from build123d import *

# Parameters (mm, degrees)
CYLINDER016_R     = 1.65
CYLINDER016_DEPTH = 50
CYLINDER017_R     = 3.25
CYLINDER017_DEPTH = 2.5
BOX005_W          = 80
BOX005_H          = 100
BOX005_DEPTH      = 9.5
CYLINDER014_R     = 22.95
CYLINDER014_DEPTH = 27
CYLINDER015_R     = 27.75
CYLINDER015_DEPTH = 40
SKETCH013_R       = 27.75
PAD001_DEPTH      = 10
SKETCH014_W       = 24
SKETCH014_H       = 14.2
POCKET013_DEPTH   = 28
SKETCH015_R       = 8.1
POCKET014_DEPTH   = 15
POCKET015_DEPTH   = 14.4
PAD003_DEPTH      = 5
PAD004_DEPTH      = 10
POCKET017_DEPTH   = 10
SKETCH022_R       = 2.6
POCKET018_DEPTH   = 4.2
SKETCH023_W       = 108.293205
SKETCH023_H       = 87.132465
POCKET019_DEPTH   = 20
SKETCH024_R       = 27.699707
PAD005_DEPTH      = 10
SKETCH025_W       = 11.3
SKETCH025_H       = 5.3
POCKET020_DEPTH   = 33
POCKET021_DEPTH   = 5.3
SKETCH027_R       = 4.253317
POCKET022_DEPTH   = 8


with BuildPart() as cylinder016:
    # Cylinder016 → Cylinder016 (new body)
    with BuildSketch(Plane(origin=(0, 50, 20), x_dir=(1, 0, 0), z_dir=(0, -1, 0))):
        Circle(CYLINDER016_R)
    extrude(amount=CYLINDER016_DEPTH)


with BuildPart() as cylinder017:
    # Cylinder017 → Cylinder017 (new body)
    with BuildSketch(Plane(origin=(0, 27.75, 20), x_dir=(1, 0, 0), z_dir=(0, -1, 0))):
        Circle(CYLINDER017_R)
    extrude(amount=CYLINDER017_DEPTH)


with BuildPart() as obj1:
    # Box005 → Box005 (new body)
    with BuildSketch(Plane(origin=(-40, 0, -1), x_dir=(1, 0, 0), z_dir=(0, 0, 1))):
        with Locations((40, 50)):
            Rectangle(BOX005_W, BOX005_H)
    extrude(amount=BOX005_DEPTH)


with BuildPart() as fusion007:
    # Cylinder014 → Cylinder014 (new body)
    with BuildSketch(Plane.XY.offset(-1)):
        Circle(CYLINDER014_R)
    extrude(amount=CYLINDER014_DEPTH)

    # Cut011: cut obj1
    add(obj1.part, mode=Mode.SUBTRACT)

    # Fusion007: union Cylinder016, Cylinder017
    add(cylinder016.part)
    add(cylinder017.part)


with BuildPart() as obj2:
    # Cylinder015 → Cylinder015 (new body)
    with BuildSketch(Plane.XY.offset(-14)):
        Circle(CYLINDER015_R)
    extrude(amount=CYLINDER015_DEPTH)

    # Cut010: cut Fusion007
    add(fusion007.part, mode=Mode.SUBTRACT)

    # Sketch013 (on Face2 of BaseFeature003) → Pad001 (new body)
    with BuildSketch(Plane(origin=(0, 0, -14), x_dir=(1, 0, 0), z_dir=(0, 0, -1))):
        Circle(SKETCH013_R)
    extrude(amount=PAD001_DEPTH)

    # Sketch014 → Pocket013 (cut)
    with BuildSketch(Plane(origin=(0, 28, 0), x_dir=(-1, 0, 0), z_dir=(0, 1, 0))):
        with Locations((0, -12.1)):
            Rectangle(SKETCH014_W, SKETCH014_H)
    extrude(amount=-POCKET013_DEPTH, mode=Mode.SUBTRACT)

    # Sketch015 (on Face6 of Pocket013) → Pocket014 (cut)
    with BuildSketch(Plane(origin=(0, 0, -24), x_dir=(1, 0, 0), z_dir=(0, 0, -1))):
        Circle(SKETCH015_R)
    extrude(amount=-POCKET014_DEPTH, mode=Mode.SUBTRACT)

    # Sketch016 (on Face6 of Pocket014) → Pocket015 (cut)
    with BuildSketch(Plane(origin=(0, 0, -19.3), x_dir=(1, 0, 0), z_dir=(0, 0, -1))):
        Polygon((0, -14.036056), (12.155581, -7.018028), (12.155581, 7.018028), (0, 14.036056), (-12.155581, 7.018028), (-12.155581, -7.018028), align=None)
    extrude(amount=-POCKET015_DEPTH, mode=Mode.SUBTRACT)

    # Sketch019 (on Face8 of Pocket015) → Pad003 (join)
    with BuildSketch(Plane.XY.offset(25)):
        with BuildLine():
            ThreePointArc((-15.553331, -22.846971), (0.028426, -27.638548), (15.600294, -22.814929))
            Line((15.600294, -22.814929), (5.918583, -80.985076))
            ThreePointArc((-5.919268, -80.980951), (-0.002091, -86), (5.918583, -80.985076))
            Line((-15.553331, -22.846971), (-5.919268, -80.980951))
        make_face()
    extrude(amount=-PAD003_DEPTH)

    # Sketch020 (on Face12 of Pad003) → Pad004 (join)
    with BuildSketch(Plane.XY.offset(25)):
        with BuildLine():
            ThreePointArc((-5.898869, -81.096969), (0.071542, -85.999573), (5.92335, -80.955994))
            Line((11.272496, -48.593121), (5.92335, -80.955994))
            ThreePointArc((-11.235042, -48.601794), (0.019223, -49.883466), (11.272496, -48.593121))
            Line((-11.235042, -48.601794), (-5.898869, -81.096969))
        make_face()
    extrude(amount=PAD004_DEPTH)

    # Sketch021 (on Face10 of Pad004) → Pocket017 (cut)
    with BuildSketch(Plane(origin=(0, 0, 20), x_dir=(1, 0, 0), z_dir=(0, 0, -1))):
        with BuildLine():
            ThreePointArc((17.426701, 54.194258), (-0.181494, 56.926923), (-17.771906, 54.082038))
            Line((-17.771906, 54.082038), (-17.771906, 91.276634))
            Line((17.426701, 91.276634), (-17.771906, 91.276634))
            Line((17.426701, 54.194258), (17.426701, 91.276634))
        make_face()
    extrude(amount=-POCKET017_DEPTH, mode=Mode.SUBTRACT)

    # Sketch022 (on Face33 of Pocket017) → Pocket018 (cut)
    with BuildSketch(Plane.XY.offset(35)):
        with Locations((0, -67.25)):
            Circle(SKETCH022_R)
    extrude(amount=-POCKET018_DEPTH, mode=Mode.SUBTRACT)

    # Sketch023 (on Face6 of Pocket018) → Pocket019 (cut)
    with BuildSketch(Plane(origin=(0, 0, -24), x_dir=(1, 0, 0), z_dir=(0, 0, -1))):
        with Locations((-3.019794, 5.274049)):
            Rectangle(SKETCH023_W, SKETCH023_H)
    extrude(amount=-POCKET019_DEPTH, mode=Mode.SUBTRACT)

    # Sketch024 (on Face2 of Pocket019) → Pad005 (join)
    with BuildSketch(Plane(origin=(0, 0, -4), x_dir=(1, 0, 0), z_dir=(0, 0, -1))):
        Circle(SKETCH024_R)
    extrude(amount=PAD005_DEPTH)

    # Sketch025 → Pocket020 (cut)
    with BuildSketch(Plane.XZ.offset(-33)):
        with Locations((0, -8.627069)):
            Rectangle(SKETCH025_W, SKETCH025_H)
    extrude(amount=POCKET020_DEPTH, mode=Mode.SUBTRACT)

    # Sketch026 → Pocket021 (cut)
    with BuildSketch(Plane.XY.offset(-6)):
        Polygon((5.65, -3.262029), (5.65, 3.262029), (0, 6.524058), (-5.65, 3.262029), (-5.65, -3.262029), (0, -6.524058), align=None)
    extrude(amount=-POCKET021_DEPTH, mode=Mode.SUBTRACT)

    # Sketch027 (on Face16 of Pocket021) → Pocket022 (cut)
    with BuildSketch(Plane(origin=(0, 0, -14), x_dir=(1, 0, 0), z_dir=(0, 0, -1))):
        Circle(SKETCH027_R)
    extrude(amount=-POCKET022_DEPTH, mode=Mode.SUBTRACT)


solid = obj2.part
Could you check a few things on this model? Use its own coordinates, in mm. A direction names the side the tool comes from. Give positions to 0.01 mm unless a question says otherwise; leave off trailing zeros. Order: outer loops, then holes, each group sorted by start corner. A loop starts at its lowest first (then second) coordinate and runs counter-clockwise, first axis right, second up.
Item 1: I need wall thicknesses on line 1 (Z direction, x = 0, y = 24.2); line 2 (Z direction, x = 0, y = 26.9); line 3 (X direction, y = 0, z = -12.3). Which ranges of each line are inside material? Lowest first, please.
Item 2: If we section it at D-D, the plane y = -78.5: Write out the boundary of the cut face in (x, z), plus the area to 3 significant figures.
Item 3: For faces 1 (the face through (-3.247, 26.518, 20.143)), 2 (the face through (0, -63, 35)), 3 (the face through (0, 9, 8.5)), 4 (the face through (14.891, -23.356, -8.93)), which set-ups out of +Z, -Z, +X, -X, +Y, -Y let a thin tool reach every point of the face, with its end or its side?
Item 4: If we section it at B-B, the plane y = -9.5: Write out the boundary of the cut face in (x, z).
Item 5: If we mould it in two halves opening along X, with no side actions, what happens to faces 5 (the face through (0, 14, -5.977)), 6 (the face through (12.86, -39.27, 22.54)), 7 (the face through (-6.02, 27.09, 11.21))? For each: pulls with the +X half, pulls with the -X half, needs draft (parallel to the pull), parting line crosses it, or undercut.
Item 6: If we section it at A-A, the plane x = 24.5: Write out the boundary of the cut face in (y, z), plus the area to 3 significant figures.
Item 7: I'm going to push flat-ended pins straight in: pin 1 (2 mm diameter, centred on x = 0, z = 19, fed in from +Y); pin 2 (3.5 mm diameter, centred on x = 1.5, y = 17, fed in from +Z); pin 3 (10 mm diameter, centred on x = -17.5, z = -6.5, fed in from -Y). Where does each tip first touch, or does it pass through?
Values:
1. line 1: z = -14 to -11.28, -5.98 to 18.35, 21.65 to 26
1. line 2: z = -14 to -11.28, -5.98 to 16.75, 23.25 to 26
1. line 3: x = -27.7 to -4.25, 4.25 to 27.7
2. outline: (-6.33, 30) - (6.33, 30) - (6.33, 35) - (-6.33, 35) - close
2. area: 63.3 mm2
3. face 1: +Y
3. face 2: +Z, +X, -X, +Y, -Y
3. face 3: +Z
3. face 4: -Z
4. outline: (-26.07, -4) - (-26.02, -4) - (-26.02, -14) - (26.02, -14) - (26.02, -4) - (26.07, -4) - (26.07, 26) - (20.89, 26) - (20.89, -1) - (-20.89, -1) - (-20.89, 26) - (-26.07, 26) - close
5. face 5: undercut
5. face 6: pulls with the +X half
5. face 7: parting line crosses it
6. outline: (-13.03, -4) - (-12.92, -4) - (-12.92, -14) - (12.92, -14) - (12.92, -4) - (13.03, -4) - (13.03, 26) - (-13.03, 26) - close
6. area: 1,040 mm2
7. pin 1: stops at y = 25.25
7. pin 2: stops at z = 8.5
7. pin 3: stops at y = -24.72
